Input: part model. Units: mm. Frame: model coordinates. A direction names the side the tool comes from. Give positions to 0.01 mm unless a question says otherwise; leave off trailing zeros. Loops run counter-clockwise (first coordinate to the right, second up) from the corner with the lowest first, then second, coordinate; pieces in that order, holes last.
from build123d import *

# Parameters (mm, degrees)
SKETCH1_W           = 56
SKETCH1_H           = 46.5
BOSS_EXTRUDE1_DEPTH = 2.5
SKETCH2_W           = 51
SKETCH2_H           = 41.5
SKETCH2_W_2         = 46
SKETCH2_H_2         = 36.5
BOSS_EXTRUDE2_DEPTH = 2.5
CUT_EXTRUDE1_DEPTH  = 2.5
FILLET1_R           = 2


with BuildPart() as part:
    # Sketch1 → Boss-Extrude1 (new body)
    with BuildSketch(Plane(origin=(0, 0, 0), x_dir=(1, 0, 0), z_dir=(0, 1, 0))):
        Rectangle(SKETCH1_W, SKETCH1_H)
    extrude(amount=BOSS_EXTRUDE1_DEPTH)

    # Sketch2 → Boss-Extrude2 (add)
    with BuildSketch(Plane.XZ):
        Rectangle(SKETCH2_W, SKETCH2_H)
        Rectangle(SKETCH2_W_2, SKETCH2_H_2, mode=Mode.SUBTRACT)
    extrude(amount=BOSS_EXTRUDE2_DEPTH)

    # Sketch3 → Cut-Extrude1 (cut)
    with BuildSketch(Plane.XZ.offset(2.5)):
        Polygon((-3, 20.75), (3, 20.75), (3, 3), (25.5, 3), (25.5, -3), (3, -3), (3, -20.75), (-3, -20.75), (-3, -3), (-25.5, -3), (-25.5, 3), (-3, 3), align=None)
    extrude(amount=-CUT_EXTRUDE1_DEPTH, mode=Mode.SUBTRACT)

    # Fillet1
    fillet1_edges = [part.edges().sort_by_distance(p)[0] for p in [
        (-3, 0, 19.5),
        (3, 0, 19.5),
        (24.25, 0, 3),
        (24.25, 0, -3),
        (3, 0, -19.5),
        (-3, 0, -19.5),
        (-24.25, 0, -3),
        (-24.25, 0, 3),
    ]]
    fillet(fillet1_edges, radius=FILLET1_R)


solid = part.part
(1) Cut plane B-B (z = 5.5). Return the cut outline in (x, y).
Values follow:
outline: (-28, 0) - (-25.5, 0) - (-25.5, -2.5) - (-23, -2.5) - (-23, 0) - (23, 0) - (23, -2.5) - (25.5, -2.5) - (25.5, 0) - (28, 0) - (28, 2.5) - (-28, 2.5) - close
(2) Pin query (flat end, axial travel): pin 1 Ø4 at (x, z) = (8.5, 2) entering from -Y; pin 2 Ø0.6 at (x, y) = (-23.5, -2) entering from +Z; pin 3 Ø0.8 at (x, y) = (-8.5, -2) entering from -Z. Return the tip coordinate at first contact, or that it passes through.
Values follow:
pin 1: stops at y = 0
pin 2: stops at z = 20.75
pin 3: stops at z = -20.75
(3) Cut plane A-A (y = -1.05). Return the cut outline in (x, z), and give its area (3 significant figures).
Values follow:
outline: (-25.5, -20.75) - (-2.76, -20.75) - (-2.76, -18.25) - (-23, -18.25) - (-23, -2.76) - (-25.5, -2.76) - close; (-25.5, 2.76) - (-23, 2.76) - (-23, 18.25) - (-2.76, 18.25) - (-2.76, 20.75) - (-25.5, 20.75) - close; (2.76, -20.75) - (25.5, -20.75) - (25.5, -2.76) - (23, -2.76) - (23, -18.25) - (2.76, -18.25) - close; (2.76, 18.25) - (23, 18.25) - (23, 2.76) - (25.5, 2.76) - (25.5, 20.75) - (2.76, 20.75) - close
area: 382 mm2
(4) Ray query, probe 1 along Z at (x, y) = (-18, -1.25); probe 2 along X at (y, z) = (-1.9, 14.5); probe 3 along Z at (x, y) = (23.5, -2.3). Return the intervals inside material, ascending.
Values follow:
probe 1: z = -20.75 to -18.25, 18.25 to 20.75
probe 2: x = -25.5 to -23, 23 to 25.5
probe 3: z = -20.75 to -3, 3 to 20.75
(5) Reachability of faces 4 (the cylindrical face through (-24.23, -0.57, 2.4)), 5 (the flat face through (23, -1, -10)), 6 (the flat face through (-13, -1, -20.75)) from +Z, -Z, +X, -X, +Y, -Y: full face, straight path, thin tool, end or side. Return the list, or none.
Values follow:
face 4: +X, -X, -Y
face 5: -Y
face 6: -Z, +X, -X, -Y
(6) Mould query, pull axis Z, two halves, no side actions, for faces 1 (the flat face through (-18, -2.5, 19)), 2 (the cylindrical face through (24.27, -0.57, 2.4)), 3 (the flat face through (0, 1, 23.25)). Classes: +Z half, -Z half, draft (parallel to the pull), parting line (faces both ways), or undercut.
Values follow:
face 1: draft
face 2: undercut
face 3: +Z half
(7) Cut plane C-C (x = -10). Return the cut outline in (y, z), and give its area (3 significant figures).
Values follow:
outline: (-2.5, -20.75) - (0, -20.75) - (0, -23.25) - (2.5, -23.25) - (2.5, 23.25) - (0, 23.25) - (0, 20.75) - (-2.5, 20.75) - (-2.5, 18.25) - (0, 18.25) - (0, -18.25) - (-2.5, -18.25) - close
area: 129 mm2
